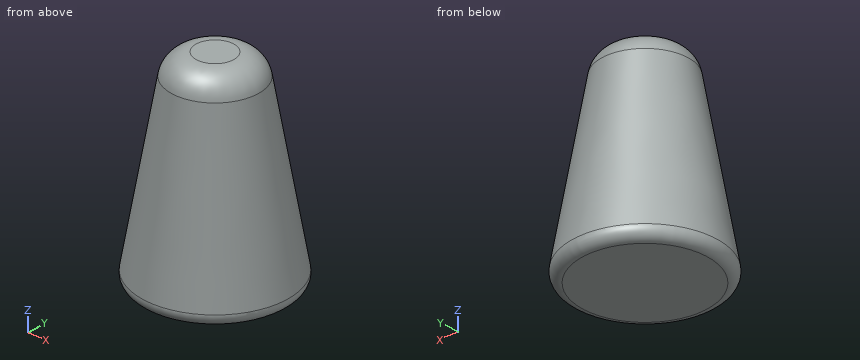
from build123d import *

# Parameters (mm, degrees)
FILLET014_R = 2
FILLET015_R = 5


with BuildPart() as part:
    # Cone014 → Cone014 (revolve)
    with BuildSketch(Plane(origin=(10, -18, 16), x_dir=(1, 0, 0), z_dir=(0, -1, 0))):
        Polygon((0, 0), (15, 0), (8, 40), (0, 40), align=None)
    revolve(axis=Axis((10, -18, 16), (0, 0, 1)))

    # Fillet014
    fillet014_edges = [part.edges().sort_by_distance(p)[0] for p in [
        (-5, -18, 16),
    ]]
    fillet(fillet014_edges, radius=FILLET014_R)


with BuildPart() as part_1:
    # Fillet014 placement: moved
    add(part.part.moved(Location((0, 0, 14))))

    # Fillet015
    fillet015_edges = [part_1.edges().sort_by_distance(p)[0] for p in [
        (2, -18, 70),
    ]]
    fillet(fillet015_edges, radius=FILLET015_R)


with BuildPart() as part_2:
    # Fillet015 placement: moved
    add(part_1.part.moved(Location((-1, 0, 0))))


solid = part_2.part
The model under review builds one solid part; all positions refer to its coordinate system, in mm. Coordinates: 2 decimals unless noted, no trailing zeros. Write each loop counter-clockwise with the first axis right and the second up, starting at its lowest first coordinate (ties: lowest second). Pieces come first, ordered by that corner, then holes. Notation, with made-up numbers: M -27.75,2 L 27.25,2 A22 ccw 27.25,8 Z; hole C 46,27.25 d3. An arc over 180 degrees is marked long. Put each result on its own line as item: value.
1) Clearance check with flat-ended pins moving along their axes: pin 1 Ø10 at (x, z) = (-0.5, 52) entering from +Y; pin 2 Ø6 at (x, z) = (4.5, 43) entering from -Y; pin 3 Ø3 at (y, z) = (-15.5, 61) entering from -X. State where each tip first meets the part, or that it passes through.
Computed:
pin 1: stops at y = -7.6
pin 2: stops at y = -30.88
pin 3: stops at x = -0.65
2) Wall thickness on probe 1 along X at (y, z) = (-29, 40); probe 2 along Y at (x, z) = (7.5, 64); probe 3 along X at (y, z) = (-28, 41): over which ranges is each line inside the solid? List them lowest first. Write a range as [from, to].
Computed:
probe 1: x = [1.61, 16.39]
probe 2: y = [-26.92, -9.08]
probe 3: x = [0.58, 17.42]
3) Add section B-B on z = 56. Give the boundary of the cut face in (x, y), then the cut area to 3 significant figures.
Computed:
outline: C 9,-18 d20.9
area: 343 mm2
4) Add section A-A on z = 60. Give the boundary of the cut face in (x, y), then the cut area to 3 significant figures.
Computed:
outline: C 9,-18 d19.5
area: 299 mm2
